Model file for the job. Use its own axes, mm. A direction names the side the tool comes from. Coordinates: 2 decimals unless noted, no trailing zeros. Write each loop counter-clockwise with the first axis right and the second up, starting at its lowest first coordinate (ties: lowest second). Pieces come first, ordered by that corner, then holes. Notation, with made-up numbers: (2, 12) - (42, 12) arc R20 cw to (42, 21) - close; hole circle Ø5 at (26.5, 35). An arc over 180 degrees is marked (long way). Put each result on its own line as item: value. Start each with the question number.
1. Pull direction Z, two halves, no side cores. Call faces 1 (the face through (0, -1, 65)), 2 (the face through (21, -19, -55)), 3 (the face through (0, -21, 1)), 4 (the face through (22.5, -1.25, -55.07)): released by +Z, released by -Z, zero draft, split by the parting line, or undercut.
2. Drop flat-ended pins along their axis: P1, Ø12, axis at x = -4.5, z = 38, coming from the +Y side; P2, Ø2.5, axis at x = -21.5, z = 55.5, coming from the +Y side. Give the stop position or say it passes through.
3. Saw through at D-D, the plane z = 55. Write the cut outline in (x, y).
4. Which spindle directions (+Z, -Z, +X, -X, +Y, -Y) get a long thin tool onto all of the face, cutting with end or side? Do faces 5 (the face through (-19.5, -1.25, 54.93)), 6 (the face through (30, 19, 0)). Say none if no direction does.
5. Saw through at A-A, the plane y = -17. Give the number of separate pieces and of enclosed holes in the cut face, plus the area to 3 significant figures.
6. Saw through at C-C, the plane x = 9. Write the cut outline in (y, z), plus the area to 3 significant figures.
7. Drill centre lines: L1, parallel to X at y = -8, z = -55; L2, parallel to Z at x = 21, y = -1; L3, parallel to Z at x = 5.5, y = 4. Where is each one in solid material? Low to high. Write a range as from..to.
Autodesk Inventor part; units mm, degrees
sketch "Cuerpo" plane through (0, 0, 0) normal (0, 1, 0) x (-1, 0, 0)
  line L0 (0, -91.5799) -> (0, 91.5799)
  line L1 (-43.9799, 0) -> (43.9799, 0)
  line L2 (29, -65) -> (-29, -65)
  line L3 (-31, -63) -> (-31, 63)
  line L4 (-29, 65) -> (29, 65)
  line L5 (31, 63) -> (31, -63)
  arc A0 (29, -65) -> (31, -63) centre (29, -63) ccw
  arc A1 (-31, -63) -> (-29, -65) centre (-29, -63) ccw
  arc A2 (31, 63) -> (29, 65) centre (29, 63) ccw
  arc A3 (-29, 65) -> (-31, 63) centre (-29, 63) ccw
  circle A4 centre (21, -55) radius 1.5
  circle A5 centre (21, -55) radius 3
  circle A6 centre (-21, -55) radius 1.5
  circle A7 centre (-21, -55) radius 3
  circle A8 centre (21, 55) radius 1.5
  circle A9 centre (21, 55) radius 3
  circle A10 centre (-21, 55) radius 3
  circle A11 centre (-21, 55) radius 1.5
  line L6 (29, -63) -> (-29, -63)
  line L7 (-29, -63) -> (-29, 63)
  line L8 (-29, 63) -> (29, 63)
  line L9 (29, 63) -> (29, -63)
  point P0 (0, 0)
  point P1 (31, -65)
  point P2 (-31, 65)
  dimension "d0" = 31
  dimension "d1" = 65
  dimension "d2" = 31
  dimension "d3" = 65
  dimension "d4" = 2
  dimension "d5" = 10
  dimension "d6" = 10
  dimension "d7" = 10
  dimension "d8" = 10
  dimension "d9" = 10
  dimension "d10" = 10
  dimension "d11" = 10
  dimension "d12" = 10
  dimension "d13" = 3
  dimension "d14" = 6
  dimension "d15" = 3
  dimension "d16" = 6
  dimension "d17" = 3
  dimension "d18" = 6
  dimension "d19" = 6
  dimension "d20" = 3
extrude "Extrusión1" add sketch "Cuerpo" along normal mid plane 38 contours L2 A1 L3 L1 L7 L6 L0 | L0 L6 L9 L1 L5 A0 L2 | L8 L7 L1 L3 A3 L4 L0 | L0 L4 A2 L5 L1 L9 L8 | A5 | A7 | A9 | A10
ref_plane "Plano de trabajo1" through (0, -19, 0) normal (0, 1, 0) x (-1, 0, 0)
sketch "Boceto2" plane through (0, -19, 0) normal (0, 1, 0) x (-1, 0, 0)
  line L0 (-29, -65) -> (29, -65)
  line L1 (31, -63) -> (31, 63)
  line L2 (29, 65) -> (-29, 65)
  line L3 (-31, 63) -> (-31, -63)
  arc A0 (-31, -63) -> (-29, -65) centre (-29, -63) ccw
  arc A1 (29, -65) -> (31, -63) centre (29, -63) ccw
  arc A2 (-29, 65) -> (-31, 63) centre (-29, 63) ccw
  arc A3 (31, 63) -> (29, 65) centre (29, 63) ccw
  line L4 (-43.9799, 0) -> (43.9799, 0)
  line L5 (0, -91) -> (0, 91)
  point P0 (0, 0)
  dimension "d24" = 2
  dimension "d34" = 65
  dimension "d35" = 65
  dimension "d36" = 31
extrude "Base" add sketch "Boceto2" against normal blind 2
sketch "Boceto3" plane through (29, 19, -65) normal (0, 0, -1) x (-1, 0, 0)
  line L0 (58, -40) -> (0, -40)
  line L1 (-2, -40) -> (-2, 0)
  circle A0 centre (29, -17) radius 2.5
  point P0 (29, -19)
  dimension "d27" = 23
  dimension "d28" = 31
  dimension "d29" = 5
extrude "Extrusión3" cut sketch "Boceto3" against normal blind 200
sketch "Boceto4" plane through (-21, 19, 55) normal (0, 1, 0) x (1, 0, 0)
  point P0 (21, 55)
sketch "Boceto5" plane through (-21, 19, 55) normal (0, 1, 0) x (1, 0, 0)
  circle A0 centre (0, 0) radius 1.5
  circle A1 centre (0, 0) radius 3
  circle A2 centre (0, 110) radius 1.5
  circle A3 centre (0, 110) radius 3
  circle A4 centre (42, 110) radius 1.5
  circle A5 centre (42, 110) radius 3
  circle A6 centre (42, 0) radius 1.5
  circle A7 centre (42, 0) radius 3
  point P0 (21, 55)
extrude "Extrusión4" cut sketch "Boceto5" against normal blind 2 contours A1 | A2 | A3 | A4 | A5 | A7
equation "\"d15\" = d13"
equation "\"d16\" = d14"
equation "\"d17\" = d13"
equation "\"d18\" = d14"
equation "\"d19\" = d14"
equation "\"d20\" = d13"
properties part number "Resistencia_Cuerpo" material "PVC, no plastificado"
Final values:
1. face 1: released by +Z
1. face 2: undercut
1. face 3: zero draft
1. face 4: undercut
2. P1: stops at y = -19
2. P2: stops at y = 17
3. outline: (-31, -21) - (31, -21) - (31, 19) - (29, 19) - (29, -19) - (24, -19) - (24, 17) - (22.5, 17) - (22.5, -19) - (19.5, -19) - (19.5, 17) - (18, 17) - (18, -19) - (-18, -19) - (-18, 17) - (-19.5, 17) - (-19.5, -19) - (-22.5, -19) - (-22.5, 17) - (-24, 17) - (-24, -19) - (-29, -19) - (-29, 19) - (-31, 19) - close
4. face 5: +Y
4. face 6: +Z, -Z, +X, -X, +Y
5. separate pieces: 5
5. enclosed holes: 5
5. area: 833 mm²
6. outline: (-21, -65) - (19, -65) - (19, -63) - (-19, -63) - (-19, 63) - (19, 63) - (19, 65) - (-21, 65) - close
6. area: 412 mm²
7. L1: x = -31..-29, -24..-22.5, -19.5..-18, 18..19.5, 22.5..24, 29..31
7. L2: z = -65..-63, -58..-56.5, -53.5..-52, 52..53.5, 56.5..58, 63..65
7. L3: z = -65..-63, 63..65
